from build123d import *

# Parameters (mm, degrees)
SKETCH1_R           = 0.4445
BOSS_EXTRUDE1_DEPTH = 2.159
SKETCH1_3_R         = 1.9558
BOSS_EXTRUDE2_DEPTH = 3.8608
SKETCH2_R           = 1.27
CUT_EXTRUDE1_DEPTH  = 17.503394679


with BuildPart() as part:
    # Sketch1 → Boss-Extrude1 (new body)
    with BuildSketch(Plane.XY):
        with BuildLine():
            Line((1.9558, -13.97), (1.9558, 0))
            ThreePointArc((1.9558, 0), (0, -1.9558), (-1.9558, 0))
            Line((-1.9558, 0), (-1.9558, -13.97))
            ThreePointArc((-1.9558, -13.97), (0, -15.9258), (1.9558, -13.97))
        make_face()
        with Locations((0, -10.4648)):
            Circle(SKETCH1_R, mode=Mode.SUBTRACT)
        with Locations((0, -7.9248)):
            Circle(SKETCH1_R, mode=Mode.SUBTRACT)
        with Locations((0, -13.0048)):
            Circle(SKETCH1_R, mode=Mode.SUBTRACT)
        with Locations((0, -5.3848)):
            Circle(SKETCH1_R, mode=Mode.SUBTRACT)
        with Locations((0, -2.8448)):
            Circle(SKETCH1_R, mode=Mode.SUBTRACT)
    extrude(amount=-BOSS_EXTRUDE1_DEPTH)

    # Sketch1<3> → Boss-Extrude2 (add)
    with BuildSketch(Plane.XY):
        Circle(SKETCH1_3_R)
    extrude(amount=-BOSS_EXTRUDE2_DEPTH)

    # Sketch2 → Cut-Extrude1 (cut, through all)
    with BuildSketch(Plane(origin=(0, 0, -3.8608), x_dir=(-1, 0, 0), z_dir=(0, 0, -1))):
        Circle(SKETCH2_R)
    extrude(amount=-CUT_EXTRUDE1_DEPTH, mode=Mode.SUBTRACT)


solid = part.part
Verification items for the finished model (mm, model axes). A direction names the side the tool comes from. Coordinates: 2 decimals unless noted, no trailing zeros. Order: outer loops, then holes, each group sorted by start corner. A loop starts at its lowest first (then second) coordinate and runs counter-clockwise, first axis right, second up. Notation, with made-up numbers: M 56.25,-9 L 81.25,-9 A25 cw 81.25,21 Z; hole C 89.25,61 d1. An arc over 180 degrees is marked long. Write each question's results on one line, items separated by ' | '.
1) Section check D-D on y = 0.5. Record the cut outline in (x, z).
Solved:
outline: M -1.89,-3.86 L -1.17,-3.86 L -1.17,0 L -1.89,0 Z; M 1.17,-3.86 L 1.89,-3.86 L 1.89,0 L 1.17,0 Z
2) Section check C-C on z = -1.45. Record the cut outline in (x, y), plus the area to 3 significant figures.
Solved:
outline: M -1.96,-13.97 A1.96 ccw 1.96,-13.97 L 1.96,0 A1.96 ccw -1.96,0 Z; hole C 0,0 d2.54; hole C 0,-13 d0.89; hole C 0,-10.46 d0.89; hole C 0,-7.92 d0.89; hole C 0,-5.38 d0.89; hole C 0,-2.84 d0.89 | area: 58.5 mm²
3) Gauge pin test, flat ends, axial feed: pin 1 Ø2 at (x, y) = (0, -11) entering from -Z; pin 2 Ø1.5 at (x, y) = (0, 0) entering from -Z; pin 3 Ø1.5 at (x, y) = (-1, -0.5) entering from -Z; pin 4 Ø1.5 at (x, z) = (1, -1.5) entering from -Y. Record the tip position at first contact, or that the pin passes through.
Solved:
pin 1: stops at z = -2.16 | pin 2: passes through | pin 3: stops at z = -3.86 | pin 4: stops at y = -15.91
4) Release check for a two-part mould opening along X. For faces 1 (the face through (0, -9.6, -2.159)), 2 (the face through (-0.058, -2.404, -1.064)), 3 (the face through (0.205, -10.859, -1.064)), 4 (the face through (-1.956, -7, -1)) record: pulls with the +X half, pulls with the -X half, needs draft (parallel to the pull), parting line crosses it, or undercut.
Solved:
face 1: needs draft | face 2: undercut | face 3: undercut | face 4: pulls with the -X half
5) Section check A-A on x = 0. Give the number of separate pieces and of enclosed holes in the cut face, plus the area to 3 significant figures.
Solved:
separate pieces: 7 | enclosed holes: 0 | area: 25.9 mm²
6) Access from +Z, -Z, +X, -X, +Y, -Y to the whole of each face (thin tool, end or side, straight path). Record for faces 5 (the face through (-0.328, -12.704, -1.064)), 6 (the face through (-0.25, 1.94, -2.33)).
Solved:
face 5: +Z, -Z | face 6: -Z
7) Section check B-B on x = -1.1. Record the cut outline in (y, z).
Solved:
outline: M -15.59,-2.16 L -1.62,-2.16 L -1.62,-3.86 L -0.63,-3.86 L -0.63,0 L -15.59,0 Z; M 0.63,-3.86 L 1.62,-3.86 L 1.62,0 L 0.63,0 Z
8) Scan lines: line 1 along Z through (x, y) = (-0.4, -14); line 2 along Y through (x, z) = (0, -2.4); line 3 along X through (y, z) = (0.5, -0.65). Record each from-to range of solid material in increasing order. Write a range as [from, to].
Solved:
line 1: z = [-2.16, 0] | line 2: y = [-1.96, -1.27], [1.27, 1.96] | line 3: x = [-1.89, -1.17], [1.17, 1.89]
